Part model, mm, in its own coordinate system. A direction names the side the tool comes from. Coordinates: 2 decimals unless noted, no trailing zeros. Loops run counter-clockwise (first coordinate to the right, second up) from the corner with the lowest first, then second, coordinate; pieces in that order, holes last. Notation, with made-up numbers: (-23, -19) -> (-9, -19) arc R19 cw to (-9, -6) -> close; hole circle Ø6 at (71, 67.5). An arc over 180 degrees is marked (long way). One line per item, written item: value. Start each with the question number.
from build123d import *

# Parameters (mm, degrees)
BOSS_EXTRUDE1_DEPTH   = 38
BOSS_EXTRUDE1_2_DEPTH = 38
SKETCH2_W             = 42.5
SKETCH2_H             = 5.7
BOSS_EXTRUDE2_DEPTH   = 2
BOSS_EXTRUDE3_DEPTH   = 18
SKETCH4_W             = 42.5
SKETCH4_H             = 40
BOSS_EXTRUDE4_DEPTH   = 2
SKETCH5_W             = 37.1
SKETCH5_H             = 11.85
CUT_EXTRUDE1_DEPTH    = 81.281509747
SKETCH6_W             = 2
SKETCH6_H             = 21
BOSS_EXTRUDE6_DEPTH   = 50
BOSS_EXTRUDE7_DEPTH   = 42.5


with BuildPart() as part:
    # Sketch1 → Boss-Extrude1 (new body)
    with BuildSketch(Plane(origin=(0, 0, 0), x_dir=(1, 0, 0), z_dir=(0, 1, 0))):
        Polygon((-62.898983402, -26.09346473), (-62.898983402, -24.39346473), (-62.198983402, -24.39346473), (-62.198983402, -22.39346473), (-64.898983402, -22.39346473), (-64.898983402, -28.09346473), (-62.198983402, -28.09346473), (-62.198983402, -26.09346473), align=None)
    extrude(amount=BOSS_EXTRUDE1_DEPTH)



with BuildPart() as body_2:
    # Sketch1 → Boss-Extrude1 2 (new body)
    with BuildSketch(Plane(origin=(0, 0, 0), x_dir=(1, 0, 0), z_dir=(0, 1, 0))):
        Polygon((-25.098983402, -22.39346473), (-25.098983402, -24.39346473), (-24.398983402, -24.39346473), (-24.398983402, -26.09346473), (-25.098983402, -26.09346473), (-25.098983402, -28.09346473), (-22.398983402, -28.09346473), (-22.398983402, -22.39346473), align=None)
    extrude(amount=BOSS_EXTRUDE1_2_DEPTH)


with BuildPart() as part_1:
    add(part.part)

    add(body_2.part)  # Boss-Extrude2 merges body 2
    # Sketch2 → Boss-Extrude2 (add)
    with BuildSketch(Plane(origin=(0, 0, 0), x_dir=(1, 0, 0), z_dir=(0, 1, 0))):
        with Locations((-43.648983402, -25.24346473)):
            Rectangle(SKETCH2_W, SKETCH2_H)
    extrude(amount=-BOSS_EXTRUDE2_DEPTH)

    # Sketch3 → Boss-Extrude3 (add)
    with BuildSketch(Plane(origin=(0, 0, 22.39346473), x_dir=(-1, 0, 0), z_dir=(0, 0, -1))):
        Polygon((64.898983402, 38), (62.198983402, 38), (62.198983402, 0), (25.098983402, 0), (25.098983402, 38), (22.398983402, 38), (22.398983402, -2), (64.898983402, -2), align=None)
    extrude(amount=BOSS_EXTRUDE3_DEPTH)

    # Sketch4 → Boss-Extrude4 (add)
    with BuildSketch(Plane(origin=(0, 0, 4.39346473), x_dir=(-1, 0, 0), z_dir=(0, 0, -1))):
        with Locations((43.648983402, 18)):
            Rectangle(SKETCH4_W, SKETCH4_H)
    extrude(amount=BOSS_EXTRUDE4_DEPTH)

    # Sketch5 → Cut-Extrude1 (cut, through all)
    with BuildSketch(Plane(origin=(0, 0, 0), x_dir=(1, 0, 0), z_dir=(0, 1, 0))):
        with Locations((-43.648983402, -10.31846473)):
            Rectangle(SKETCH5_W, SKETCH5_H)
    extrude(amount=-CUT_EXTRUDE1_DEPTH, mode=Mode.SUBTRACT)

    # Sketch6 → Boss-Extrude6 (add)
    with BuildSketch(Plane(origin=(0, 0, 2.39346473), x_dir=(-1, 0, 0), z_dir=(0, 0, -1))):
        with Locations((27.148983402, 8.5)):
            Rectangle(SKETCH6_W, SKETCH6_H)
        with Locations((60.148983402, 8.5)):
            Rectangle(SKETCH6_W, SKETCH6_H)
    extrude(amount=BOSS_EXTRUDE6_DEPTH)

    # Sketch7 → Boss-Extrude7 (add)
    with BuildSketch(Plane.XZ.offset(2)):
        Polygon((-59.148983402, -47.60653527), (-61.148983402, -47.60653527), (-61.148983402, -49.60653527), (-26.148983402, -49.60653527), (-26.148983402, -47.60653527), (-28.148983402, -47.60653527), align=None)
    extrude(amount=-BOSS_EXTRUDE7_DEPTH)


solid = part_1.part
1) Slice it at B-B (x = -60). Give the cut face in (y, z).
2) Tool access for faces 5 (the flat face through (-24.399, 19, 25)), 6 (the flat face through (-26.149, 10, -24)), 7 (the flat face through (-27, 19, -22)): list every direction of +Z, -Z, +X, -X, +Y, -Y with a clear straight run to the whole face (end or side of a thin tool).
3) Slice it at D-D (y = 34). Give the cut face in (x, z), then the cut area to 3 significant figures.
4) Pin check, flat tips, straight feed: pin 1 Ø12 at (x, z) = (-56.5, 19) entering from +Y; pin 2 Ø3.5 at (x, z) = (-46.5, 22) entering from +Y; pin 3 Ø21 at (y, z) = (28.5, -21) entering from -X. Stop position of each tip, or through.
5) Pull direction Z, two halves, no side cores. Call faces 1 (the flat face through (-64.899, 18, 15)), 2 (the flat face through (-60, 19, -22)), 3 (the flat face through (-44, 19, -49.607)), 4 (the flat face through (-44, -1, 28.093)): +Z half, -Z half, draft (parallel to the pull), parting line (faces both ways), or undercut.
6) Slice it at C-C (y = 15). Give the cut face in (x, z).
7) Probe line 1 (Z direction, x = -35, y = 6); line 2 (X direction, y = 28.5, z = 9); line 3 (X direction, y = 16, z = -38.5). List the from-to ranges inside material, lowest first. Write a range as from..to.
8) Slice it at A-A (z = -10.5). Give the cut face in (x, y), then the cut area to 3 significant figures.
Check sheet entries:
1. outline: (-2, -49.61) -> (40.5, -49.61) -> (40.5, -47.61) -> (19, -47.61) -> (19, 2.39) -> (38, 2.39) -> (38, 4.39) -> (-2, 4.39) -> close; (-2, 16.24) -> (0, 16.24) -> (0, 28.09) -> (-2, 28.09) -> close
2. face 5: +Y
2. face 6: -Z, +X, +Y, -Y
2. face 7: +X, -X, +Y
3. outline: (-64.9, 2.39) -> (-22.4, 2.39) -> (-22.4, 28.09) -> (-25.1, 28.09) -> (-25.1, 26.09) -> (-24.4, 26.09) -> (-24.4, 24.39) -> (-25.1, 24.39) -> (-25.1, 4.39) -> (-62.2, 4.39) -> (-62.2, 24.39) -> (-62.9, 24.39) -> (-62.9, 26.09) -> (-62.2, 26.09) -> (-62.2, 28.09) -> (-64.9, 28.09) -> close; (-61.15, -49.61) -> (-26.15, -49.61) -> (-26.15, -47.61) -> (-61.15, -47.61) -> close
3. area: 281 mm^2
4. pin 1: stops at y = 38
4. pin 2: stops at y = 0
4. pin 3: stops at x = -61.15
5. face 1: draft
5. face 2: undercut
5. face 3: -Z half
5. face 4: +Z half
6. outline: (-64.9, 2.39) -> (-61.15, 2.39) -> (-61.15, -49.61) -> (-26.15, -49.61) -> (-26.15, 2.39) -> (-22.4, 2.39) -> (-22.4, 28.09) -> (-25.1, 28.09) -> (-25.1, 26.09) -> (-24.4, 26.09) -> (-24.4, 24.39) -> (-25.1, 24.39) -> (-25.1, 4.39) -> (-62.2, 4.39) -> (-62.2, 24.39) -> (-62.9, 24.39) -> (-62.9, 26.09) -> (-62.2, 26.09) -> (-62.2, 28.09) -> (-64.9, 28.09) -> close; hole (-59.15, -47.61) -> (-28.15, -47.61) -> (-28.15, 2.39) -> (-59.15, 2.39) -> close
7. line 1: z = -49.61..-47.61, 2.39..4.39
7. line 2: x = -64.9..-62.2, -25.1..-22.4
7. line 3: x = -61.15..-59.15, -28.15..-26.15
8. outline: (-61.15, -2) -> (-59.15, -2) -> (-59.15, 19) -> (-61.15, 19) -> close; (-28.15, -2) -> (-26.15, -2) -> (-26.15, 19) -> (-28.15, 19) -> close
8. area: 84.0 mm^2
